Check sheet for the modelled part. Datum: model origin and axes. Units: mm. A direction names the side the tool comes from. Round coordinates to 2 decimals unless told otherwise and drop trailing zeros. Loops run counter-clockwise (first coordinate to the right, second up) from the corner with the lowest first, then second, coordinate; pieces in that order, holes last. Notation, with made-up numbers: (5, -39.5) - (62, -39.5) arc R22 ccw to (62, -7.5) - close; hole circle Ø9 at (-17.5, 63.5). An arc over 180 degrees is marked (long way). Put each result on its own line as item: value. Start each with the question number.
Item 1: Section check A-A, the plane z = 5. Record the cut outline in (x, y).
Item 2: Draft check along Y on faces 1 (the cylindrical face through (28.595, 70.545, 1.479)), 2 (the flat face through (51.182, 13, 6)), 3 (the flat face through (39.054, 43.519, 1.726)). Enter one of: pulls with the +Y half, pulls with the -Y half, needs draft (parallel to the pull), parting line crosses it, or undercut.
Item 3: Tool access check on faces 4 (the flat face through (36, 58, 8)), 5 (the flat face through (36, 15.877, 6)), 6 (the flat face through (51.182, 60, 6)), 7 (the flat face through (33.31, 43.52, 1.73)), 8 (the flat face through (21.182, 59, 6)). Record the directions out of +Z, -Z, +X, -X, +Y, -Y that give a thin tool (end or side, any length) a straight path to the whole face; none if there is none.
Item 4: Gauge pin test, flat ends, axial feed: pin 1 Ø3 at (x, y) = (36.18, 36.38) entering from -Z; pin 2 Ø1 at (y, z) = (56.5, 2) entering from -X; pin 3 Ø2 at (y, z) = (11.5, 6.5) entering from -X. Record the tip position at first contact, or that the pin passes through.
Item 5: Section check B-B, the plane z = 1.5. Record the cut outline in (x, y), and give its area (3 significant figures).
Item 6: Material ranges on line 1 along Y through (x, z) = (35.5, 5.25); line 2 along Y through (x, z) = (39.5, 6.5), recorded low to high.
Solid Edge part; units mm, degrees
sketch "Sketch1" plane through (0, 0, 0) normal (0, 0, 1) x (1, 0, 0)
  circle A0 centre (36.1822, 36.3769) radius 35
  circle A1 centre (36.1822, 36.3769) radius 35
extrude "Protrusion1" add sketch "Sketch1" along normal blind 4
sketch "Sketch2" plane through (36.1822, 36.3769, 4) normal (0, 0, 1) x (1, 0, 0)
  circle A0 centre (14, 0) radius 1.75
  circle A1 centre (-14, 0) radius 1.75
  circle A2 centre (0, 0) radius 1
extrude "Cutout1" cut sketch "Sketch2" against normal through all
sketch "Sketch3" plane through (36.1822, 36.3769, 0) normal (0, 0, -1) x (0, -1, 0)
  line L0 (0.473, 3.72) -> (14, 2)
  arc A0 (14, 2) -> (14, -2) centre (14, 0) cw
  line L1 (0.473, -3.72) -> (14, -2)
  line L2 (0.473, -3.72) -> (-0.473, -3.72)
  line L3 (-0.473, -3.72) -> (-14, -2)
  arc A1 (-14, 2) -> (-14, -2) centre (-14, 0) ccw
  line L4 (-0.473, 3.72) -> (-14, 2)
  line L5 (-0.473, 3.72) -> (0.473, 3.72)
  dimension "D1" = 14
extrude "Enlèvement_matière_2" cut sketch "Sketch3" against normal blind 3.5
sketch "Sketch4" plane through (36.1822, 36.3769, 4) normal (0, 0, 1) x (0, 1, 0)
  line L0 (20.5, -15) -> (25.5, -15)
  line L1 (25.5, -15) -> (25.5, 15)
  line L2 (25.5, 15) -> (20.5, 15)
  line L3 (20.5, 15) -> (20.5, -15)
  line L4 (-25.5, -15) -> (-20.5, -15)
  line L5 (-20.5, -15) -> (-20.5, 15)
  line L6 (-20.5, 15) -> (-25.5, 15)
  line L7 (-25.5, 15) -> (-25.5, -15)
  dimension "D1" = 25.5
  dimension "D2" = 25.5
extrude "Ajout_matière_2" add sketch "Sketch4" along normal blind 4
fillet "Congé_1" radius 0.25 2 edges at (36.1822, 56.8769, 8) (36.1822, 15.8769, 8)
fillet "Congé_2" radius 3 2 edges at (36.1822, 61.8769, 8) (36.1822, 10.8769, 8)
fillet "Congé_3" radius 3 2 edges at (36.1822, 61.8769, 4) (36.1822, 10.8769, 4)
fillet "Congé_4" radius 1 1 edges at (1.1822, 36.3769, 4)
properties part number "AC_1.02"
Check result:
1. outline: (21.18, 10.46) - (51.18, 10.46) - (51.18, 15.88) - (21.18, 15.88) - close; (21.18, 56.88) - (51.18, 56.88) - (51.18, 62.3) - (21.18, 62.3) - close
2. face 1: parting line crosses it
2. face 2: needs draft
2. face 3: undercut
3. face 4: +Z, +X, -X, +Y, -Y
3. face 5: +Z, +X, -X
3. face 6: +Z, +X, +Y, -Y
3. face 7: -Z
3. face 8: +Z, -X, +Y, -Y
4. pin 1: z = 3.5
4. pin 2: x = 7.2
4. pin 3: x = 21.18
5. outline: circle Ø70 at (36.18, 36.38); hole circle Ø3.5 at (22.18, 36.38); hole (32.46, 35.9) - (34.18, 22.38) arc R2 ccw to (38.18, 22.38) - (39.9, 35.9) - (39.9, 36.85) - (38.18, 50.38) arc R2 ccw to (34.18, 50.38) - (32.46, 36.85) - close; hole circle Ø3.5 at (50.18, 36.38)
5. area: 3,650 mm²
6. line 1: 10.66 to 15.88, 56.88 to 62.1
6. line 2: 11.28 to 15.88, 56.88 to 61.47
